Autodesk Inventor part; units mm, degrees
ref_plane "YZ Plane" through (0, 0, 0) normal (1, 0, 0) x (0, 1, 0)
ref_plane "XZ Plane" through (0, 0, 0) normal (0, 1, 0) x (-1, 0, 0)
ref_plane "XY Plane" through (0, 0, 0) normal (0, 0, 1) x (1, 0, 0)
sketch "Sketch1" plane through (0, 0, 0) normal (0, 1, 0) x (-1, 0, 0)
  line L0 (25, 100) -> (-25, 100)
  line L1 (-25, 100) -> (-25, -100)
  line L2 (-25, -100) -> (25, -100)
  line L3 (25, -100) -> (25, 100)
  line L4 (25, 100) -> (-25, -100) construction
  line L5 (-25, 100) -> (25, -100) construction
  point P0 (0, 0)
  dimension "d0" = 200
  dimension "d1" = 50
extrude "Extrusion1" add sketch "Sketch1" along normal blind 3
sketch "Sketch2" plane through (0, 3, 0) normal (0, 1, 0) x (1, 0, 0)
  line L0 (0, 0) -> (25, 0) construction
  line L1 (25, -100) -> (25, 100)
  line L2 (25, -92) -> (-15.0756, -92) construction
  circle A0 centre (17.5, -92) radius 2
  circle A1 centre (5.5, -92) radius 2
  line L3 (-25, -100) -> (25, -100)
  circle A2 centre (17.5, 92) radius 2
  circle A3 centre (5.5, 92) radius 2
  dimension "d4" = 4
  dimension "d5" = 4
  dimension "d6" = 12
  dimension "d7" = 8
  dimension "d10" = 7.5
extrude "Extrusion2" cut sketch "Sketch2" against normal blind 5
sketch "Sketch3" plane through (0, 3, 0) normal (0, 1, 0) x (1, 0, 0)
  line L0 (19, -85) -> (31, -85)
  line L1 (31, -85) -> (31, 85)
  line L2 (31, 85) -> (19, 85)
  line L3 (19, 85) -> (19, -85)
  line L4 (25, -100) -> (25, 100)
  line L5 (19, -85) -> (31, 85) construction
  line L6 (31, -85) -> (19, 85) construction
  point P0 (0, 0)
  point P1 (25, 0)
  dimension "d11" = 170
  dimension "d12" = 12
extrude "Extrusion3" add sketch "Sketch3" against normal blind 3
sketch "Sketch4" plane through (0, 3, 0) normal (0, 1, 0) x (1, 0, 0)
  line L0 (25, -100) -> (25, 100)
  line L1 (31, 85) -> (25, 85)
  circle A0 centre (26, -75) radius 2
  line L2 (25, -85) -> (31, -85)
  line L3 (31, -85) -> (31, 85)
  point P0 (0, 0)
  dimension "d15" = 4
  dimension "d16" = 10
  dimension "d17" = 5
extrude "Extrusion4" cut sketch "Sketch4" against normal blind 5 contours A0 L0 | L0 A0
pattern_linear "Rectangular Pattern1" count 6 spacing 30 along (0, 0, -1) of "Extrusion4"
fillet "Fillet1" radius 10 2 edges at (-25, 1.5, -100) (-25, 1.5, 100)
sketch "Sketch5" plane through (0, 3, 0) normal (0, 1, 0) x (1, 0, 0)
  line L0 (31, 85) -> (25, 85)
  line L1 (32.3908, 88) -> (-29, 88)
  line L2 (-29, 88) -> (-29, -105)
  line L3 (-29, -105) -> (32.3908, -105)
  line L4 (32.3908, -105) -> (32.3908, 84.997)
  line L5 (32.3908, 84.997) -> (32.3908, 88)
  line L6 (25, 100) -> (-15, 100)
  point P0 (0, 0)
  dimension "d31" = 12
extrude "Extrusion5" cut sketch "Sketch5" against normal blind 10
sketch "Sketch6" plane through (0, 3, 0) normal (0, 1, 0) x (1, 0, 0)
  line L0 (25, 94.8) -> (30, 94.8)
  line L1 (30, 94.8) -> (30, 91)
  line L2 (30, 91) -> (25, 91)
  line L3 (25, 91) -> (25, 94.8)
  line L4 (25, 100) -> (-15, 100)
  point P0 (0, 0)
  dimension "d26" = 5.2
  dimension "d27" = 5
  dimension "d28" = 3.8
extrude "Extrusion6" add sketch "Sketch6" against normal blind 3
properties part number "Comb4"
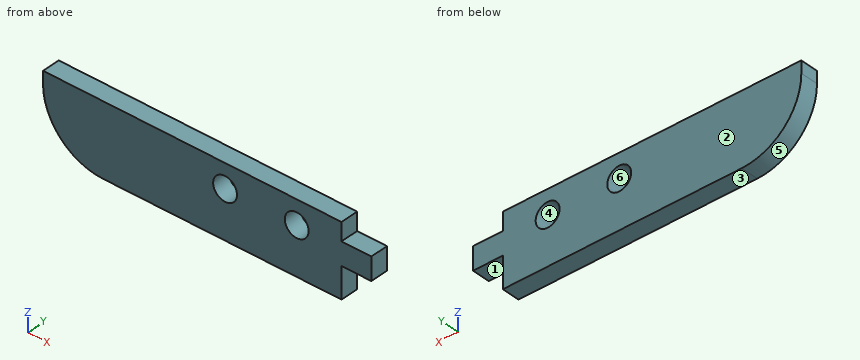
Here's how the part is built. I have some questions about the finished solid (model axes, mm). Face numbers are marked on the shaded views. A direction names the side the tool comes from. Round coordinates to 2 decimals unless told otherwise and drop trailing zeros. Loops run counter-clockwise (first coordinate to the right, second up) from the corner with the lowest first, then second, coordinate; pieces in that order, holes last. Notation, with made-up numbers: (87, 3.25) -> (92, 3.25) arc R17 ccw to (92, 22.25) -> close; hole circle Ø8 at (23.5, 11). An arc over 180 degrees is marked (long way). Answer as CSV lines item,"result".
1. If I drill on L1, parallel to Z at x = 5.5, y = 2.3; L2, parallel to X at y = 0.65, z = -92; L3, parallel to X at y = 1.45, z = -98.75, over which ranges is the centre line in solid material (lowest first)?
Final values:
L1,"z = -100 to -94, -90 to -88"
L2,"x = -24.8 to 3.5, 7.5 to 15.5, 19.5 to 30"
L3,"x = -19.84 to 25"
2. If we section it at D-D on z = -96.75: Please give me the cut outline in (x, y).
Final values:
outline,"(-22.38, 0) -> (25, 0) -> (25, 3) -> (-22.38, 3) -> close"
3. For pin 1 (0.9 mm diameter, centred on x = 26.5, y = 1, fed in from +Z), with a flat end and sliding along its axis, tell me the tip position at first contact or that it passes through.
Final values:
pin 1,"stops at z = -91"
4. Thinking about a two-plate mould opening in X: for the marked faces 3, 4, 5 and 6, which applies, released by +X, released by -X, zero draft, split by the parting line, or undercut?
Final values:
face 3,"zero draft"
face 4,"undercut"
face 5,"released by -X"
face 6,"undercut"
5. Which directions (+Z, -Z, +X, -X, +Y, -Y) give clear straight access to the entire face, cutting with the end or side of a thin tool? Please do the marked faces 1 and 2.
Final values:
face 1,"-Z, +X, +Y, -Y"
face 2,"+Z, -Z, +X, -X, +Y"
6. If we section it at A-A on y = 1.9: Please give me the cut outline in (x, z).
Final values:
outline,"(-25, -90) arc R10 ccw to (-15, -100) -> (25, -100) -> (25, -94.8) -> (30, -94.8) -> (30, -91) -> (25, -91) -> (25, -88) -> (-25, -88) -> close; hole circle Ø4 at (5.5, -92); hole circle Ø4 at (17.5, -92)"
7. If we section it at C-C on z = -92: Please give me the cut outline in (x, y).
Final values:
outline,"(-24.8, 0) -> (3.5, 0) -> (3.5, 3) -> (-24.8, 3) -> close; (7.5, 0) -> (15.5, 0) -> (15.5, 3) -> (7.5, 3) -> close; (19.5, 0) -> (30, 0) -> (30, 3) -> (19.5, 3) -> close"
8. If we section it at B-B on x = 17.5: Please give me the cut outline in (y, z).
Final values:
outline,"(0, -100) -> (3, -100) -> (3, -94) -> (0, -94) -> close; (0, -90) -> (3, -90) -> (3, -88) -> (0, -88) -> close"
